Geometry check sheet. Reference: the model listing, model coordinates, mm. A direction names the side the tool comes from. Give positions to 0.01 mm unless a question says otherwise; leave off trailing zeros. Order: outer loops, then holes, each group sorted by start corner. A loop starts at its lowest first (then second) coordinate and runs counter-clockwise, first axis right, second up.
```python
from build123d import *

# Parameters (mm, degrees)
F4_T      = -1.524
F6_DEPTH  = 1.524
F7_DEPTH  = 1.143
F9_DEPTH  = 1.524
F10_DEPTH = 13.97
F12_DEPTH = 1.524


with BuildPart() as f3:
    # F3: sweep along a path in F0
    with BuildLine(Plane.XY) as f3_path:
        ThreePointArc((93.98, -30.48), (85.0526146906, -8.9273853094), (63.5, 0))
        Line((63.5, 0), (0, 0))
    # F2 (on plane+point) → F3 (sweep)
    with BuildSketch(Plane.XZ.offset(30.48)):
        with BuildLine():
            Line((98.4885, 0), (89.4715, 0))
            ThreePointArc((89.4715, 0), (93.98, -4.5085), (98.4885, 0))
        make_face()
    sweep(path=f3_path.line)

    # F4
    f4_openings = [f3.faces().sort_by_distance(p)[0] for p in [
        (87.501546, -6.478454, 0),
    ]]
    offset(amount=F4_T, openings=f4_openings)

    # F5 (on face) → F6 (cut, through all)
    with BuildSketch(Plane.XZ.offset(30.48)):
        with BuildLine():
            ThreePointArc((91.5035, 0), (93.98, -2.4765), (96.4565, 0))
            Line((96.4565, 0), (91.5035, 0))
        make_face()
    extrude(amount=-F6_DEPTH, mode=Mode.SUBTRACT)

    # F5 (on face) → F7 (cut)
    with BuildSketch(Plane.XZ.offset(30.48)):
        with BuildLine():
            Line((97.4725, 0), (96.4565, 0))
            ThreePointArc((96.4565, 0), (93.98, -2.4765), (91.5035, 0))
            Line((91.5035, 0), (90.4875, 0))
            ThreePointArc((90.4875, 0), (93.98, -3.4925), (97.4725, 0))
        make_face()
    extrude(amount=-F7_DEPTH, mode=Mode.SUBTRACT)

    # F8 (on face) → F9 (cut, through all)
    with BuildSketch(Plane(origin=(0, 0, 0), x_dir=(0, -1, 0), z_dir=(-1, 0, 0))):
        with BuildLine():
            ThreePointArc((-2.413, 0), (0, -2.413), (2.413, 0))
            Line((2.413, 0), (-2.413, 0))
        make_face()
    extrude(amount=-F9_DEPTH, mode=Mode.SUBTRACT)

    # F5 (on face) → F10 (join)
    with BuildSketch(Plane.XZ.offset(30.48)):
        with BuildLine():
            Line((98.4885, 0), (97.4725, 0))
            ThreePointArc((97.4725, 0), (93.98, -3.4925), (90.4875, 0))
            Line((90.4875, 0), (89.4715, 0))
            ThreePointArc((89.4715, 0), (93.98, -4.5085), (98.4885, 0))
        make_face()
    extrude(amount=F10_DEPTH)

    # F11 (on face) → F12 (join)
    with BuildSketch(Plane.XZ.offset(44.45)):
        with BuildLine():
            Line((98.4885, 0), (97.4725, 0))
            ThreePointArc((97.4725, 0), (93.98, -3.4925), (90.4875, 0))
            Line((90.4875, 0), (89.4715, 0))
            ThreePointArc((89.4715, 0), (93.98, -4.5085), (98.4885, 0))
        make_face()
        with BuildLine():
            ThreePointArc((90.4875, 0), (93.98, -3.4925), (97.4725, 0))
            Line((97.4725, 0), (95.6945, 0))
            ThreePointArc((95.6945, 0), (93.98, -1.7145), (92.2655, 0))
            Line((92.2655, 0), (90.4875, 0))
        make_face()
    extrude(amount=F12_DEPTH)


solid = f3.part
```
Q1. Thickness scan on L1, parallel to X at y = -36, z = -0.35; L2, parallel to Y at x = 58, z = -1.05; L3, parallel to X at y = -25, z = -1. Record the ranges inside material, lowest first.
Q2. Gauge pin test, flat ends, axial feed: P1, Ø1, axis at x = 66, z = -1.5, coming from the -Y side; P2, Ø2, axis at y = -16.5, z = -3.5, coming from the -X side; P3, Ø1.5, axis at x = 92.5, z = -1, coming from the +Y side. Record the tip position at first contact, or that the pin passes through.
Q3. Release check for a two-part mould opening along X. For faces 1 (the face through (31.306, 0.099, -4.507)), 2 (the face through (1.524, -0.2, -2.6)), 3 (the face through (93.881, -38.119, -4.507)) record: pulls with the +X half, pulls with the -X half, needs draft (parallel to the pull), parting line crosses it, or undercut.
Q4. Access from +Z, -Z, +X, -X, +Y, -Y to the whole of each face (thin tool, end or side, straight path). Record for faces 4 (the face through (94.018, -45.201, -1.714)), 5 (the face through (0.751, 0.053, -2.412)), 6 (the face through (94.06, -36.79, -3.49)).
Q5. Cross-section at A-A, the plane x = 38. Record the boundary of the cut face in (y, z), and give its area (3 significant figures).
Answers follow:
1. L1: x = 89.49 to 90.51, 97.45 to 98.47
1. L2: y = -4.38 to -2.79, 2.79 to 4.38
1. L3: x = 89 to 90.62, 96.34 to 97.94
2. P1: stops at y = -4.53
2. P2: stops at x = 86.07
2. P3: stops at y = -9.99
3. face 1: needs draft
3. face 2: undercut
3. face 3: parting line crosses it
4. face 4: +Z, -Y
4. face 5: +Z, -X
4. face 6: +Z
5. outline: (-4.51, 0) arc R4.51 ccw to (4.51, 0) - (2.98, 0) arc R2.98 cw to (-2.98, 0) - close
5. area: 17.9 mm2
